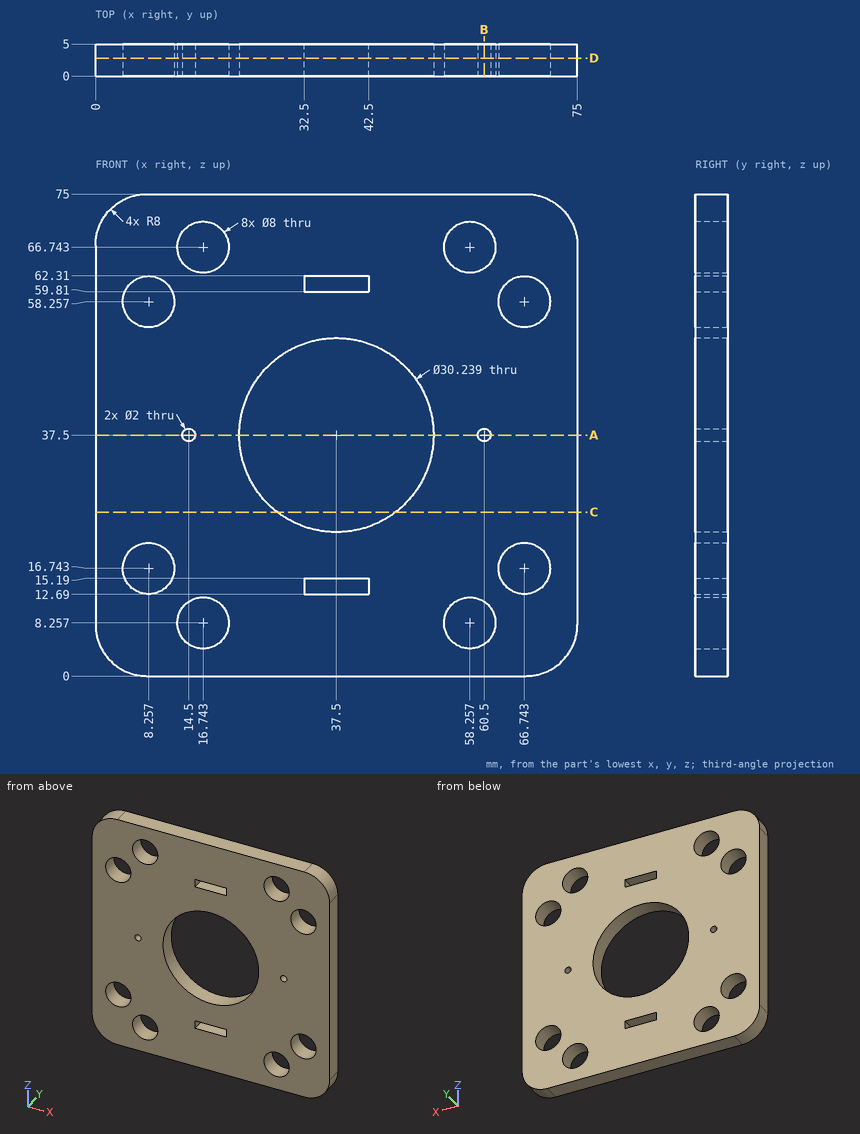
Could you check a few things on this drawing? It's one solid part, dimensions in mm from its lowest x, y, z. Give positions to 0.01 mm unless a question says otherwise; leave off trailing zeros. Order: outer loops, then holes, each group sorted by start corner. A loop starts at its lowest first (then second) coordinate and runs counter-clockwise, first axis right, second up. Notation, with made-up numbers: (19.25, 66) -> (50.25, 66) arc R19 ccw to (50.25, 98) -> close; hole circle Ø4 at (20, 35.5). An arc over 180 degrees is marked (long way). Answer in a Markdown table with one row per item. Add a question column.
Item 1: Imagine slicing it at C-C (z = 25.5). List the corners of the cut face in (x, y) for me, and give its area (3 significant figures).
Item 2: Imagine slicing it at B-B (x = 60.5). List the corners of the cut face in (y, z) for me (1 decimal).
Item 3: Imagine slicing it at D-D (y = 2.8). Count the separate pieces of the cut face and the enclosed holes in it, and give its area (3 significant figures).
Item 4: Please list where these lines run through material, in increasing order: probe 1 along X at (y, z) = (2.95, 37.5); probe 2 along Z at (x, y) = (56, 4.65) (1 decimal); probe 3 along X at (y, z) = (3.05, 65.5) (1 decimal).
Item 5: I'm going to push a flat-ended pin straight in: P1, Ø13, axis at x = 16.74, z = 8.26, coming from the +Y side. Where does the tip first touch, or does it pass through?
Item 6: Imagine slicing it at A-A (z = 37.5). List the corners of the cut face in (x, y) for me, and give its area (3 significant figures).
Result:
| question | item | result |
|---|---|---|
| 1 | outline | (0, 0) -> (28.3, 0) -> (28.3, 5) -> (0, 5) -> close; (46.7, 0) -> (75, 0) -> (75, 5) -> (46.7, 5) -> close |
| 1 | area | 283 mm2 |
| 2 | outline | (0, 0) -> (5, 0) -> (5, 4.9) -> (0, 4.9) -> close; (0, 11.6) -> (5, 11.6) -> (5, 36.5) -> (0, 36.5) -> close; (0, 38.5) -> (5, 38.5) -> (5, 63.4) -> (0, 63.4) -> close; (0, 70.1) -> (5, 70.1) -> (5, 75) -> (0, 75) -> close |
| 3 | separate pieces | 1 |
| 3 | enclosed holes | 13 |
| 3 | area | 4,390 mm2 |
| 4 | probe 1 | 0 to 13.5, 15.5 to 22.38, 52.62 to 59.5, 61.5 to 75 |
| 4 | probe 2 | 0 to 5, 11.6 to 63.4, 70 to 75 |
| 4 | probe 3 | 0 to 12.9, 20.5 to 54.5, 62.1 to 75 |
| 5 | P1 | y = 5 |
| 6 | outline | (0, 0) -> (13.5, 0) -> (13.5, 5) -> (0, 5) -> close; (15.5, 0) -> (22.38, 0) -> (22.38, 5) -> (15.5, 5) -> close; (52.62, 0) -> (59.5, 0) -> (59.5, 5) -> (52.62, 5) -> close; (61.5, 0) -> (75, 0) -> (75, 5) -> (61.5, 5) -> close |
| 6 | area | 204 mm2 |
